Drawing for the job (mm, zero at the part's lowest x, y, z). A direction names the side the tool comes from. Give positions to 0.01 mm unless a question says otherwise; leave off trailing zeros. Write each loop counter-clockwise with the first axis right and the second up, starting at its lowest first coordinate (ties: lowest second). Pieces come first, ordered by that corner, then holes.
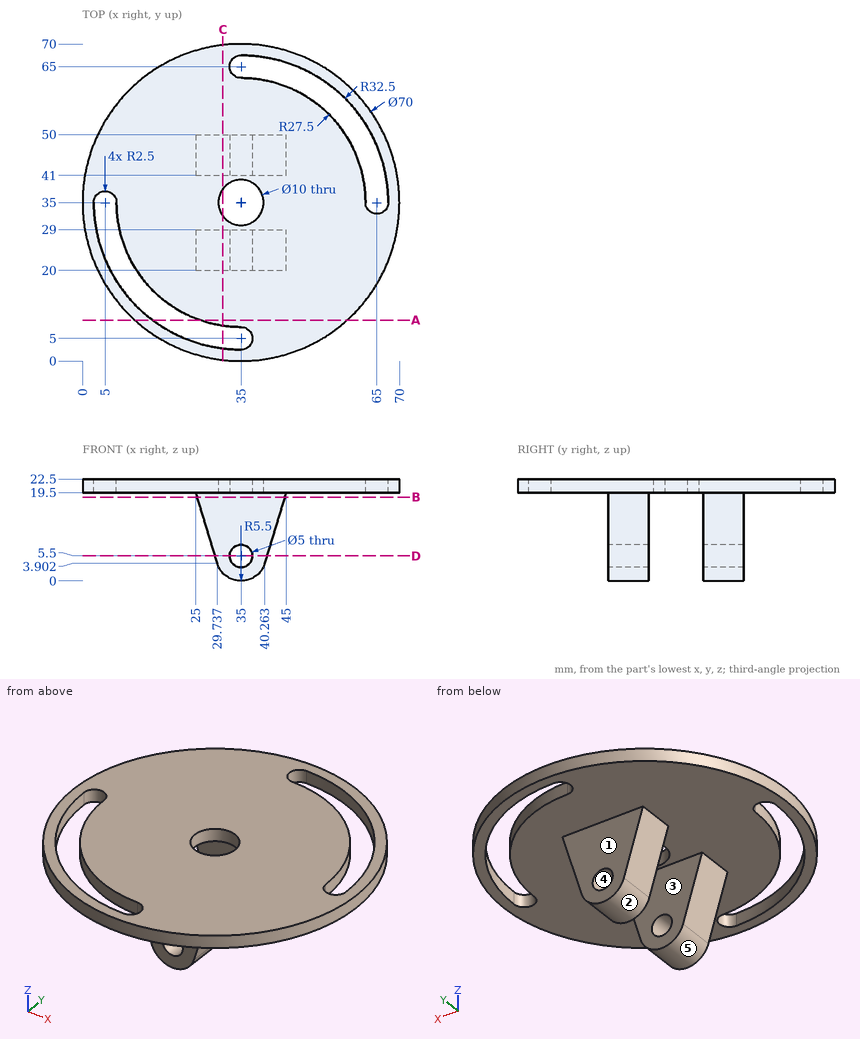
1. Pull direction Z, two halves, no side cores. Call the marked faces 3, 4 and 5: +Z half, -Z half, draft (parallel to the pull), parting line (faces both ways), or undercut.
Calculated:
face 3: draft
face 4: undercut
face 5: -Z half
2. Which spindle directions (+Z, -Z, +X, -X, +Y, -Y) get a long thin tool onto all of the face, cutting with end or side? Do the marked faces 1 and 2. Say none if no direction does.
Calculated:
face 1: -Z, +X, -X, +Y
face 2: -Z, +Y, -Y
3. Slice it at D-D, the plane z = 5.5. Write the cut outline in (x, y), and give its area (3 significant figures).
Calculated:
outline: (29.25, 20) - (32.5, 20) - (32.5, 29) - (29.25, 29) - close; (29.25, 41) - (32.5, 41) - (32.5, 50) - (29.25, 50) - close; (37.5, 20) - (40.75, 20) - (40.75, 29) - (37.5, 29) - close; (37.5, 41) - (40.75, 41) - (40.75, 50) - (37.5, 50) - close
area: 117 mm2
4. Probe probe 1 along Y at (x, z) = (35, 21.4); probe 2 along Y at (x, z) = (34.5, 13); probe 3 along Z at (x, y) = (56, 41.5). List the from-to ranges inside material, lowest first.
Calculated:
probe 1: y = 0 to 2.5, 7.5 to 30, 40 to 62.5, 67.5 to 70
probe 2: y = 20 to 29, 41 to 50
probe 3: z = 19.5 to 22.5
5. Pin check, flat tips, straight feed: P1, Ø3, axis at x = 9.5, z = 18.5, coming from the +Y side; P2, Ø6, axis at x = 38, z = 5, coming from the -Y side; P3, Ø5, axis at x = 42, y = 58.5, coming from the -Z side. Stop position of each tip, or through.
Calculated:
P1: stops at y = 60.11
P2: stops at y = 20
P3: stops at z = 19.5
6. Slice it at C-C, the plane x = 31. Write the cut outline in (y, z) (1 decimal).
Calculated:
outline: (0.2, 19.5) - (2.7, 19.5) - (2.7, 22.5) - (0.2, 22.5) - close; (7.8, 19.5) - (20, 19.5) - (20, 1.7) - (29, 1.7) - (29, 19.5) - (32, 19.5) - (32, 22.5) - (7.8, 22.5) - close; (38, 19.5) - (41, 19.5) - (41, 1.7) - (50, 1.7) - (50, 19.5) - (69.8, 19.5) - (69.8, 22.5) - (38, 22.5) - close
7. Slice it at B-B, the plane z = 18.5. Write the cut outline in (x, y).
Calculated:
outline: (25.3, 20) - (44.7, 20) - (44.7, 29) - (25.3, 29) - close; (25.3, 41) - (44.7, 41) - (44.7, 50) - (25.3, 50) - close
8. Slice it at A-A, the plane y = 9. Write the cut outline in (x, z), and give its area (3 significant figures).
Calculated:
outline: (11.57, 19.5) - (15.5, 19.5) - (15.5, 22.5) - (11.57, 22.5) - close; (26.04, 19.5) - (58.43, 19.5) - (58.43, 22.5) - (26.04, 22.5) - close
area: 109 mm2
